Read the model definition and answer for the solid it produces. Units are mm, in the model's axes. A direction names the side the tool comes from. Coordinates: 2 decimals unless noted, no trailing zeros. Loops run counter-clockwise (first coordinate to the right, second up) from the corner with the lowest first, then second, coordinate; pieces in that order, holes last. Notation, with made-up numbers: (-38.5, -34) -> (-27.5, -34) arc R23 ccw to (-27.5, -22) -> close; hole circle Ø10 at (-5, 6.25). An arc over 180 degrees is marked (long way). Answer as a JSON object with one key per item and string values. Group by question number.
Q1. The part is cut by section C-C on z = 35. Write down the section's boundary in (x, y).
Q2. For faces 1 (the cylindrical face through (19.46, 2.88, 60.73)), 2 (the flat face through (-3, 3, 0)), 3 (the flat face through (-1, -7.746, 27)), 4 (the flat face through (24.965, 3, 39)), 5 (the flat face through (-14.625, 2.9, 55.4)), determine the directions among +Z, -Z, +X, -X, +Y, -Y from which every point of the face is accessible in a straight line to the end or side of a thin tool.
Q3. The part is cut by section D-D on z = 17. Write down the section's boundary in (x, y), and give its area (3 significant figures).
Q4. Determine the mould class of faces 6 (the flat face through (-1, 13.272, 27)), 7 (the flat face through (-25.962, 3, 39)), 8 (the cylindrical face through (-62.313, 3.504, 12.522)), 9 (the cylindrical face through (-20.373, 3.42, 55.183)) for opening direction Y: released by +Y, released by -Y, zero draft, split by the parting line, or undercut.
Q5. Each of these flat-tipped pins is pushed along its axis until it touches: P1, Ø16, axis at y = 2.77, z = 50.21, coming from the +X side; P2, Ø8, axis at y = 9, z = 19, coming from the -X side; P3, Ø6, axis at x = -33.5, y = -9.5, coming from the -Z side; P4, Ø9, axis at y = 2.77, z = 50.21, coming from the +X side. Where does it stop, or does it pass through?
Q6. The part is cut by section B-B on x = -47. Write down the section's boundary in (y, z).
Q7. Straight lines are drawn through the part: line 1 along X through (y, z) = (-6, 25); line 2 along X through (y, z) = (7, 45); line 3 along X through (y, z) = (-1, 7). For each, find the intervals that lie inside material, in ascending order. Write a range as [from, to].
Q8. The part is cut by section A-A on y = -4.5. Write down the section's boundary in (x, z).
from build123d import *

# Parameters (mm, degrees)
F0_R     = 10.16
F1_DEPTH = 25.4
F2_W     = 50.927606
F2_H     = 21.017644
F3_DEPTH = 38.1
F6_DEPTH = 25.4
F7_DEPTH = 58.42
F8_R     = 5.011478
F9_DEPTH = 61.468


with BuildPart() as f1:
    # F0 (on Top) → F1 (new body)
    with BuildSketch(Plane.XY):
        with BuildLine():
            Line((41.684134, 19.716346), (-45.740517, 19.716346))
            ThreePointArc((-45.740517, 19.716346), (-62.317241, 3.139622), (-45.740517, -13.437102))
            Line((-45.740517, -13.437102), (41.684134, -13.437102))
            ThreePointArc((41.684134, -13.437102), (58.260858, 3.139622), (41.684134, 19.716346))
        make_face()
        with Locations((-45.740517, 3.139622)):
            Circle(F0_R, mode=Mode.SUBTRACT)
        with Locations((41.684134, 3.139622)):
            Circle(F0_R, mode=Mode.SUBTRACT)
    extrude(amount=F1_DEPTH)

    # F2 (on face) → F3 (join)
    with BuildSketch(Plane.XY.offset(25.4)):
        with Locations((-0.49852, 2.763115)):
            Rectangle(F2_W, F2_H)
    extrude(amount=F3_DEPTH)

    # F5 (on face) → F6 (cut)
    with BuildSketch(Plane(origin=(0, 13.271937, 0), x_dir=(-1, 0, 0), z_dir=(0, 1, 0))):
        with BuildLine():
            Line((14.624778, 63.5), (-14.100123, 63.5))
            Line((-14.100123, 63.5), (-14.100123, 41.915204))
            ThreePointArc((-14.100123, 41.915204), (0.262327, 27.552754), (14.624778, 41.915204))
            Line((14.624778, 41.915204), (14.624778, 63.5))
        make_face()
    extrude(amount=-F6_DEPTH, mode=Mode.SUBTRACT)

    # F4 (on face) → F7 (cut)
    with BuildSketch(Plane(origin=(-25.962323, 0, 0), x_dir=(0, -1, 0), z_dir=(-1, 0, 0))):
        with BuildLine():
            ThreePointArc((-13.271937, 50.746802), (-2.650794, 60.731682), (7.745707, 50.513107))
            Line((7.745707, 50.513107), (7.745707, 63.5))
            Line((7.745707, 63.5), (-13.271937, 63.5))
            Line((-13.271937, 63.5), (-13.271937, 50.746802))
        make_face()
    extrude(amount=-F7_DEPTH, mode=Mode.SUBTRACT)

    # F8 (on face) → F9 (cut)
    with BuildSketch(Plane(origin=(-25.962323, 0, 0), x_dir=(0, -1, 0), z_dir=(-1, 0, 0))):
        with Locations((-2.767733, 50.214658)):
            Circle(F8_R)
    extrude(amount=-F9_DEPTH, mode=Mode.SUBTRACT)


solid = f1.part
Final values:
{
 "1": {"outline": "(-25.96, -7.75) -> (-12.85, -7.75) -> (-12.85, 13.27) -> (-25.96, 13.27) -> close; (12.33, -7.75) -> (24.97, -7.75) -> (24.97, 13.27) -> (12.33, 13.27) -> close"},
 "2": {"face 1": "+Z, +X, -X", "face 2": "-Z, +X, -X, +Y, -Y", "face 3": "+Z, +X, -X, -Y", "face 4": "+Z, +X, +Y, -Y", "face 5": "+Z, +Y, -Y"},
 "3": {"outline": "(-45.74, -13.44) -> (41.68, -13.44) arc R16.58 ccw to (41.68, 19.72) -> (-45.74, 19.72) arc R16.58 ccw to start; hole circle Ø20.32 at (-45.74, 3.14); hole circle Ø20.32 at (41.68, 3.14)", "area": "3,110 mm2"},
 "4": {"face 6": "released by +Y", "face 7": "zero draft", "face 8": "split by the parting line", "face 9": "undercut"},
 "5": {"P1": "stops at x = 24.97", "P2": "stops at x = -62.21", "P3": "stops at z = 0", "P4": "passes through"},
 "6": {"outline": "(-13.39, 0) -> (-6.94, 0) -> (-6.94, 25.4) -> (-13.39, 25.4) -> close; (13.22, 0) -> (19.67, 0) -> (19.67, 25.4) -> (13.22, 25.4) -> close"},
 "7": {"line 1": "x = [-59.57, -50.18], [-41.3, 37.25], [46.12, 55.51]", "line 2": "x = [-25.96, -14.62], [14.1, 24.97]", "line 3": "x = [-61.79, -55.02], [-36.46, 32.41], [50.96, 57.74]"},
 "8": {"outline": "(-60.45, 0) -> (-52.44, 0) -> (-52.44, 25.4) -> (-60.45, 25.4) -> close; (-39.04, 0) -> (34.99, 0) -> (34.99, 25.4) -> (24.97, 25.4) -> (24.97, 57.82) -> (14.1, 57.82) -> (14.1, 41.92) arc R14.36 cw to (-14.62, 41.92) -> (-14.62, 57.82) -> (-25.96, 57.82) -> (-25.96, 25.4) -> (-39.04, 25.4) -> close; (48.38, 0) -> (56.4, 0) -> (56.4, 25.4) -> (48.38, 25.4) -> close"}
}
